from build123d import *

# Parameters (mm, degrees)
SKETCH1_R           = 1.5
BOSS_EXTRUDE1_DEPTH = 12.5
SKETCH2_R           = 2.5
BOSS_EXTRUDE2_DEPTH = 1
FILLET1_R           = 0.25
BOSS_EXTRUDE4_START = -4.5
SKETCH4_R           = 2.5
BOSS_EXTRUDE4_DEPTH = 1
CHAMFER2_SIZE       = 1


with BuildPart() as part:
    # Sketch1 → Boss-Extrude1 (new body)
    with BuildSketch(Plane.XY):
        Circle(SKETCH1_R)
    extrude(amount=BOSS_EXTRUDE1_DEPTH)

    # Sketch2 → Boss-Extrude2 (add)
    with BuildSketch(Plane.XY.offset(12.5)):
        Circle(SKETCH2_R)
    extrude(amount=-BOSS_EXTRUDE2_DEPTH)

    # Fillet1
    fillet1_edges = [part.edges().sort_by_distance(p)[0] for p in [
        (-1.5, 0, 0),
    ]]
    fillet(fillet1_edges, radius=FILLET1_R)

    # Sketch4 → Boss-Extrude4 (add)
    with BuildSketch(Plane.XY.offset(12.5).offset(BOSS_EXTRUDE4_START)):
        Circle(SKETCH4_R)
    extrude(amount=-BOSS_EXTRUDE4_DEPTH)

    # Chamfer2
    chamfer2_edges = [part.edges().sort_by_distance(p)[0] for p in [
        (-1.5, 0, 8),
    ]]
    chamfer(chamfer2_edges, length=CHAMFER2_SIZE - 0.0001)  # a hair under: the kernel refuses the full size


solid = part.part
CAD build for the part. Positions are in the model's coordinates, mm. A direction names the side the tool comes from. Round coordinates to 2 decimals unless told otherwise and drop trailing zeros. Loops run counter-clockwise (first coordinate to the right, second up) from the corner with the lowest first, then second, coordinate; pieces in that order, holes last.
(1) Two-plate mould, pull along Z, no slides. Class faces 1 (the cylindrical face through (-0.54, -2.44, 7.51)), 2 (the cylindrical face through (-1.5, 0.07, 10.23)), 3 (the flat face through (0, -2, 11.5)), 4 (the flat face through (0, -2, 7)): +Z half, -Z half, draft (parallel to the pull), parting line (faces both ways), or undercut.
(2) Drop flat-ended pins along their axis: pin 1 (2.5 mm diameter, centred on x = 1, y = 0.5, fed in from -Z); pin 2 (3 mm diameter, centred on y = 1.5, z = 4.5, fed in from -X); pin 3 (1.5 mm diameter, centred on x = 1.5, z = 8, fed in from +Y); pin 4 (2 mm diameter, centred on x = 0.5, z = 4, fed in from +Y). Give the stop position or say it passes through.
(3) Wall check: line 1 along Z through (x, y) = (0.6, -2.2); line 2 along Z through (x, y) = (0.1, 2); line 3 along Z through (x, y) = (1, 0.8). Give the ranges that are in metal, low to high.
(4) Which spindle directions (+Z, -Z, +X, -X, +Y, -Y) get a long thin tool onto all of the face, cutting with end or side? Do faces 5 (the cylindrical face through (-1.5, 0.07, 3.58)), 6 (the flat face through (0, 0, 12.5)). Say none if no direction does.
(5) Cut at C-C (z = 11.75). Give the cut face in (x, y).
(6) Cut at D-D (z = 1.75). Give the cut face in (x, y), plus the area to 3 significant figures.
Findings below:
1. face 1: draft
1. face 2: undercut
1. face 3: undercut
1. face 4: -Z half
2. pin 1: stops at z = 0
2. pin 2: stops at x = -1.5
2. pin 3: stops at y = 2.38
2. pin 4: stops at y = 1.5
3. line 1: z = 7 to 8.22, 11.5 to 12.5
3. line 2: z = 7 to 8.5, 11.5 to 12.5
3. line 3: z = 0 to 12.5
4. face 5: -Z
4. face 6: +Z, +X, -X, +Y, -Y
5. outline: circle Ø5 at (0, 0)
6. outline: circle Ø3 at (0, 0)
6. area: 7.07 mm2
